Here's how the part is built. I have some questions about the finished solid (model axes, mm). Face numbers are marked on the shaded views. A direction names the side the tool comes from. Give positions to 0.01 mm unless a question says otherwise; leave off trailing zeros. Write each loop counter-clockwise with the first axis right and the second up, starting at its lowest first coordinate (ties: lowest second). Pieces come first, ordered by that corner, then holes. Notation, with made-up numbers: (-29.75, 49) -> (-25.75, 49) arc R16 cw to (-25.75, 74) -> close; hole circle Ø1 at (21.25, -36.5). An arc over 180 degrees is marked (long way). Return JSON: item names as keys, results as strings.
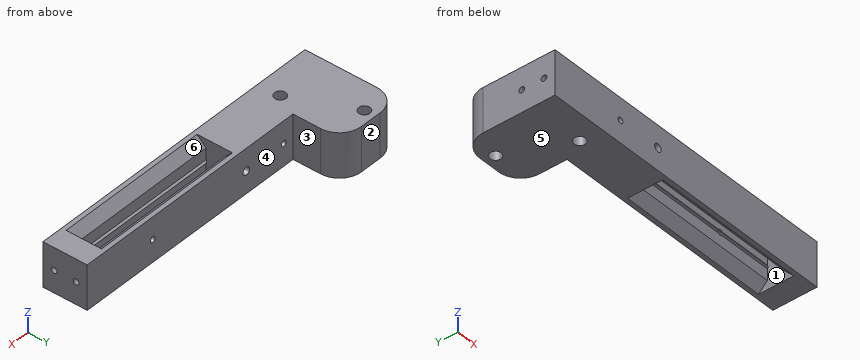
Autodesk Inventor part; units mm, degrees
ref_plane "YZ Plane" through (0, 0, 0) normal (1, 0, 0) x (0, 1, 0)
ref_plane "XZ Plane" through (0, 0, 0) normal (0, 1, 0) x (-1, 0, 0)
ref_plane "XY Plane" through (0, 0, 0) normal (0, 0, 1) x (1, 0, 0)
sketch "Sketch1" plane through (0, 0, 0) normal (1, 0, 0) x (0, 1, 0)
  line L0 (12.3116, 18.9917) -> (-13.0884, 18.9917)
  line L1 (-13.0884, 18.9917) -> (-13.0884, -6.4083)
  line L2 (-13.0884, -6.4083) -> (12.3116, -6.4083)
  line L3 (12.3116, -6.4083) -> (12.3116, 18.9917)
  point P0 (0, 0)
  dimension "d0" = 25.4
  dimension "d1" = 25.4
extrude "Extrusion1" add sketch "Sketch1" along normal blind 177.8
sketch "Sketch5" plane through (177.8, 0, 0) normal (1, 0, 0) x (0, 0, -1)
  line L0 (-18.9917, -13.0884) -> (6.4083, -13.0884)
  line L1 (-18.9917, 12.3116) -> (-18.9917, -13.0884)
  point P0 (0, 0)
  point P1 (-6.2917, 5.9616)
  point P2 (-6.2917, -6.7384)
  dimension "d31" = 6.35
  dimension "d32" = 19.05
  dimension "d33" = 12.7
  dimension "d34" = 12.7
hole "Hole4" at (177.8, 5.9616, 6.2917) at (177.8, -6.7384, 6.2917) direction (-1, 0, 0) diameter 3.302 end through all
sketch "Sketch8" plane through (0, 12.3116, 18.9917) normal (0, 1, 0) x (1, 0, 0)
  line L0 (0, 25.4) -> (38.1, 25.4)
  line L1 (38.1, 25.4) -> (38.1, 0)
  line L2 (38.1, 0) -> (0, 0)
  line L3 (0, 0) -> (0, 25.4)
  line L4 (0, 25.4) -> (0, 0)
  line L5 (0, 25.4) -> (177.8, 25.4)
  line L6 (0, 0) -> (177.8, 0)
  point P0 (0, 18.9917)
  dimension "d60" = 0
  dimension "d61" = 38.1
  dimension "d62" = 0
  dimension "d63" = 0
extrude "Extrusion2" add sketch "Sketch8" along normal blind 28.575
fillet "Fillet1" radius 12.7 2 edges at (38.1, 40.8866, 6.2917) (0, 40.8866, 6.2917)
sketch "Sketch9" plane through (0, -13.0884, 18.9917) normal (0, 0, 1) x (1, 0, 0)
  line L0 (0, 41.275) -> (0, 0)
  line L1 (12.7, 53.975) -> (25.4, 53.975)
  line L2 (38.1, 25.4) -> (177.8, 25.4)
  point P0 (0, 13.0884)
  point P1 (15.875, 47.625)
  dimension "d67" = 15.875
  dimension "d137" = 22.225
hole "Hole7" at (15.875, 34.5366, 18.9917) direction (0, 0, -1) diameter 6.477 end through all
sketch "Sketch10" plane through (0, -13.0884, 18.9917) normal (0, 0, 1) x (1, 0, 0)
  line L0 (0, 0) -> (177.8, 0)
  line L1 (0, 41.275) -> (0, 0)
  point P0 (0, 13.0884)
  point P1 (31.75, 12.7)
  dimension "d76" = 12.7
  dimension "d77" = 31.75
hole "Hole8" at (31.75, -0.3884, 18.9917) direction (0, 0, -1) diameter 6.477 end through all
sketch "Sketch11" plane through (177.8, 12.3116, 18.9917) normal (0, 1, 0) x (1, 0, 0)
  line L0 (-177.8, 25.4) -> (-177.8, 0)
  line L1 (-139.7, 0) -> (0, 0)
  point P0 (-177.8, 18.9917)
  point P1 (-107.95, 12.7)
  dimension "d85" = 69.85
  dimension "d86" = 12.7
hole "Hole9" at (69.85, 12.3116, 6.2917) direction (0, -1, 0) diameter 4.4958 end through all
sketch "Sketch12" plane through (177.8, 0, 0) normal (1, 0, 0) x (0, 0, -1)
  line L0 (-18.9917, 9.7716) -> (-18.9917, -10.5484)
  line L1 (-18.9917, -10.5484) -> (-13.9117, -5.4684)
  line L2 (-13.9117, -5.4684) -> (1.3283, -5.4684)
  line L3 (1.3283, -5.4684) -> (6.4083, -10.5484)
  line L4 (6.4083, -10.5484) -> (6.4083, 9.7716)
  line L5 (6.4083, 9.7716) -> (1.3283, 4.6916)
  line L6 (1.3283, 4.6916) -> (-13.9117, 4.6916)
  line L7 (-13.9117, 4.6916) -> (-18.9917, 9.7716)
  line L8 (-18.9917, 12.3116) -> (-18.9917, -13.0884)
  line L9 (-18.9917, -13.0884) -> (6.4083, -13.0884)
  dimension "d103" = 20.32
  dimension "d104" = 5.08
  dimension "d105" = 5.08
  dimension "d106" = 5.08
  dimension "d107" = 25.4
  dimension "d108" = 5.08
  dimension "d109" = 0
  dimension "d110" = 0
  dimension "d111" = 0
  dimension "d112" = 2.54
extrude "Extrusion3" cut sketch "Sketch12" against normal blind 101.6
sketch "Sketch13" plane through (177.8, 0, 0) normal (1, 0, 0) x (0, 0, -1)
  line L0 (-18.9917, 12.3116) -> (6.4083, 12.3116)
  line L1 (6.4083, 12.3116) -> (6.4083, -13.0884)
  line L2 (6.4083, -13.0884) -> (-18.9917, -13.0884)
  line L3 (-18.9917, -13.0884) -> (-18.9917, 12.3116)
  line L4 (6.4083, 9.7716) -> (6.4083, -10.5484)
  line L5 (-18.9917, -13.0884) -> (6.4083, -13.0884)
  point P0 (0, 0)
  dimension "d115" = 25.4
  dimension "d116" = 25.4
  dimension "d117" = 0
  dimension "d118" = 0
extrude "Extrusion4" add sketch "Sketch13" against normal blind 12.7
sketch "Sketch14" plane through (177.8, 0, 0) normal (1, 0, 0) x (0, 0, -1)
  arc A0 (-5.2368, 4.6916) -> (-7.3467, 4.6916) centre (-6.2917, 5.9616) ccw
  arc A1 (-7.3467, -5.4684) -> (-5.2368, -5.4684) centre (-6.2917, -6.7384) ccw
  point P0 (0, 0)
hole "Hole10" at (177.8, 5.9616, 6.2917) at (177.8, -6.7384, 6.2917) direction (-1, 0, 0) diameter 3.302 end through all
sketch "Sketch15" plane through (177.8, 12.3116, 18.9917) normal (0, 1, 0) x (1, 0, 0)
  line L0 (-139.7, 25.4) -> (0, 25.4)
  line L1 (-139.7, 0) -> (-139.7, 25.4)
  point P0 (-177.8, 18.9917)
  point P1 (-133.35, 12.7)
  dimension "d128" = 12.7
  dimension "d129" = 6.35
hole "Hole11" at (44.45, 12.3116, 6.2917) direction (0, -1, 0) diameter 3.302 end through all
sketch "Sketch16" plane through (177.8, 12.3116, 18.9917) normal (0, 1, 0) x (1, 0, 0)
  line L0 (-12.7, 20.32) -> (-101.6, 20.32)
  circle A0 centre (-107.95, 12.7) radius 2.2479
  line L1 (-139.7, 0) -> (0, 0)
  point P0 (-177.8, 18.9917)
  point P1 (-44.45, 12.7)
  dimension "d138" = 63.5
  dimension "d139" = 12.7
hole "Hole12" at (133.35, 12.3116, 6.2917) direction (0, -1, 0) diameter 3.302 depth 12.2936 tip angle 118.188
properties part number "BackTopBeams"
1. Which directions (+Z, -Z, +X, -X, +Y, -Y) give clear straight access to the entire face, cutting with the end or side of a thin tool? Please do the marked faces 4, 5 and 6.
Taken from the geometry:
{"face 4": "+Z, -Z, +X, +Y", "face 5": "-Z, +X, -X, +Y, -Y", "face 6": "+Z"}
2. Suppose I cut it at C-C, the plane x = 137. List the corners of the cut face in (y, z) for me.
Taken from the geometry:
{"outline": "(-13.09, -6.41) -> (-10.55, -6.41) -> (-5.47, -1.33) -> (-5.47, 5.24) arc R1.65 cw (long way) to (-5.47, 7.35) -> (-5.47, 13.91) -> (-10.55, 18.99) -> (-13.09, 18.99) -> close; (4.69, -1.33) -> (9.77, -6.41) -> (12.31, -6.41) -> (12.31, 18.99) -> (9.77, 18.99) -> (4.69, 13.91) -> (4.69, 7.35) arc R1.65 cw (long way) to (4.69, 5.24) -> close"}
3. If we mould it in two halves opening along X, with no side actions, what happens to the marked faces 1, 2 and 3? For each: released by +X, released by -X, zero draft, split by the parting line, or undercut.
Taken from the geometry:
{"face 1": "undercut", "face 2": "zero draft", "face 3": "released by +X"}
4. Suppose I cut it at A-A, the plane x = 69.85. List the corners of the cut face in (y, z) for me, and give its area (3 significant figures).
Taken from the geometry:
{"outline": "(-13.09, -6.41) -> (12.31, -6.41) -> (12.31, 4.04) -> (-13.09, 4.04) -> close; (-13.09, 8.54) -> (12.31, 8.54) -> (12.31, 18.99) -> (-13.09, 18.99) -> close", "area": "531 mm²"}
5. Suppose I cut it at B-B, the plane x = 31.75. List the corners of the cut face in (y, z) for me.
Taken from the geometry:
{"outline": "(-13.09, -6.41) -> (-3.63, -6.41) -> (-3.63, 18.99) -> (-13.09, 18.99) -> close; (2.85, -6.41) -> (39.19, -6.41) -> (39.19, 18.99) -> (2.85, 18.99) -> close; hole circle Ø3.3 at (-6.74, 6.29); hole circle Ø3.3 at (5.96, 6.29)"}
6. For pin 1 Ø5.5 at (x, z) = (124.5, 11.5) entering from +Y; pin 2 Ø3 at (y, z) = (-6.74, 6.29) entering from -X; pin 3 Ø1 at (x, z) = (33.5, 7) entering from +Y; pin 4 Ø1.5 at (y, z) = (21.5, 7) entering from +X, each with a flat end and sliding along its axis, tell me the tip position at first contact or that it passes through.
Taken from the geometry:
{"pin 1": "stops at y = 12.31", "pin 2": "passes through", "pin 3": "stops at y = 38.36", "pin 4": "stops at x = 38.1"}
7. If I drill on line 1 (X direction, y = -4.5, z = 1.5); line 2 (Y direction, x = 85, z = 11.5); line 3 (Y direction, x = 117, z = 5), over which ranges is the centre line in solid material (lowest first)? Write a range as [from, to].
Taken from the geometry:
{"line 1": "x = [0, 76.2], [165.1, 177.8]", "line 2": "y = [-13.09, -5.47], [4.69, 12.31]", "line 3": "y = [-13.09, -7.77], [-5.71, -5.47], [4.69, 4.93], [6.99, 12.31]"}
